```python
from build123d import *

# Parameters (mm, degrees)
F1_DEPTH = 10
F3_D     = 2
F4_R     = 4.99999
F5_R     = 3


# Not quite as in the source:
# - a fillet or chamfer is up to 0.001 mm smaller than in the source, because OpenCascade refuses the exact size
# - a feature names something its author has since deleted; it is built from what else it names


with BuildPart() as f1:
    # F0 (on Top) → F1 (new body)
    with BuildSketch(Plane.XY):
        with BuildLine():
            Line((-12.6909215784, 9.75), (-16, 9.75))
            ThreePointArc((-16, 9.75), (-14.3454607892, 9), (-12.6909215784, 9.75))
        make_face()
        Polygon((2, -22.25), (2, -12.25), (2, 12.25), (2, 22.25), (-2, 22.25), (-2, 12.25), (-16, 12.25), (-16, 9.75), (-12.6909215784, 9.75), (-2, 9.75), (-2, -9.25), (-12.6909215784, -9.25), (-16, -9.25), (-16, -12.25), (-2, -12.25), (-2, -22.25), align=None)
        with BuildLine():
            ThreePointArc((-12.6909215784, -9.25), (-14.3454607892, -8.5), (-16, -9.25))
            Line((-16, -9.25), (-12.6909215784, -9.25))
        make_face()
    extrude(amount=F1_DEPTH)

    # F3 (through all)
    with Locations(Plane(origin=(-2, 0, 0), x_dir=(0, -1, 0), z_dir=(-1, 0, 0))):
        with Locations((-17.25, 5), (17.3738710582, 5)):
            Hole(F3_D / 2)

    # F4 (radius 5 in the source; OpenCascade refuses exactly that, so slightly less here)
    f4_edges = [f1.edges().sort_by_distance(p)[0] for p in [
        (0, 22.25, 10),
        (0, -22.25, 10),
        (0, -22.25, 0),
        (0, 22.25, 0),
    ]]
    fillet(f4_edges, radius=F4_R)

    # F5
    f5_edges = [f1.edges().sort_by_distance(p)[0] for p in [
        (-2, 12.25, 5),
        (-2, -12.25, 5),
    ]]
    fillet(f5_edges, radius=F5_R)


solid = f1.part
```
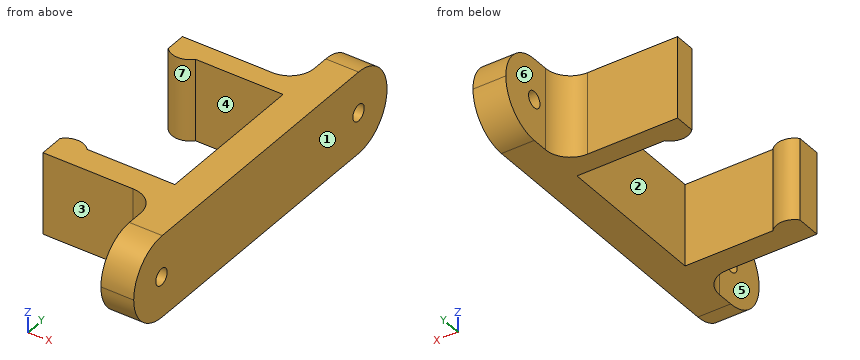
Geometry: final body of the model. Coordinates: model frame, mm. Face numbers are marked on the shaded views. A direction names the side the tool comes from. Coordinates: 2 decimals unless noted, no trailing zeros. Order: outer loops, then holes, each group sorted by start corner. A loop starts at its lowest first (then second) coordinate and runs counter-clockwise, first axis right, second up. Notation, with made-up numbers: (-11.75, 0) - (18.25, 0) arc R23 ccw to (18.25, 35) - close; hole circle Ø9 at (-22.75, -17.5). An arc over 180 degrees is marked (long way). Return JSON: item names as keys, results as strings. Group by question number.
1. Cut plane B-B (z = 2). Output: boundary loops of the cut face in (x, y), plus the area to 3 significant figures.
2. Cut plane D-D (x = -14.5). Output: boundary loops of the cut face in (y, z), plus the area to 3 significant figures.
3. Pin query (flat end, axial travel): pin 1 (4 mm diameter, centred on x = -6, z = 6.5, fed in from -Y); pin 2 (5 mm diameter, centred on x = -13, z = 3, fed in from +Y); pin 3 (3 mm diameter, centred on y = -17.37, z = 5, fed in from -X). Return the tip coordinate at first contact, or that it passes through.
4. Set-up query: the marked faces 5, 6 and 7. Return all of +Z, -Z, +X, -X, +Y, -Y with unobstructed straight access to the full face (end or side cutting, diameter ignored); none if empty.
5. Pull-direction query (Y, two-part tool) for the marked faces 1, 2, 3 and 4; classes: pulls with the +Y half, pulls with the -Y half, needs draft (parallel to the pull), parting line crosses it, or undercut.
6. Cut plane C-C (y = -3). Output: boundary loops of the cut face in (x, z), plus the area to 3 significant figures.
7. Cut plane A-A (x = -9). Output: boundary loops of the cut face in (y, z).
8. Material intervals for line 1 along Y through (x, z) = (-5.5, 4.75); line 2 along Z through (x, y) = (0.15, 17.25); line 3 along Y through (x, z) = (-14.5, 4), sorted ascending. Write a range as [from, to].
Resolved:
{
 "1": {"outline": "(-16, -12.25) - (-5, -12.25) arc R3 cw to (-2, -15.25) - (-2, -21.25) - (2, -21.25) - (2, 21.25) - (-2, 21.25) - (-2, 15.25) arc R3 cw to (-5, 12.25) - (-16, 12.25) - (-16, 9.75) arc R2.2 ccw to (-12.69, 9.75) - (-2, 9.75) - (-2, -9.25) - (-12.69, -9.25) arc R2.2 ccw to (-16, -9.25) - close", "area": "254 mm²"},
 "2": {"outline": "(-12.25, 0) - (-8.51, 0) - (-8.51, 10) - (-12.25, 10) - close; (9.01, 0) - (12.25, 0) - (12.25, 10) - (9.01, 10) - close", "area": "69.9 mm²"},
 "3": {"pin 1": "stops at y = -12.42", "pin 2": "stops at y = 12.25", "pin 3": "stops at x = -2"},
 "4": {"face 5": "+Z, -Z, -X, -Y", "face 6": "+Z, -Z, -X, +Y", "face 7": "+Z, -Z"},
 "5": {"face 1": "needs draft", "face 2": "undercut", "face 3": "pulls with the -Y half", "face 4": "undercut"},
 "6": {"outline": "(-2, 0) - (2, 0) - (2, 10) - (-2, 10) - close", "area": "40.0 mm²"},
 "7": {"outline": "(-12.25, 0) - (-9.25, 0) - (-9.25, 10) - (-12.25, 10) - close; (9.75, 0) - (12.25, 0) - (12.25, 10) - (9.75, 10) - close"},
 "8": {"line 1": "y = [-12.25, -9.25], [9.75, 12.25]", "line 2": "z = [0, 4], [6, 10]", "line 3": "y = [-12.25, -8.51], [9.01, 12.25]"}
}
